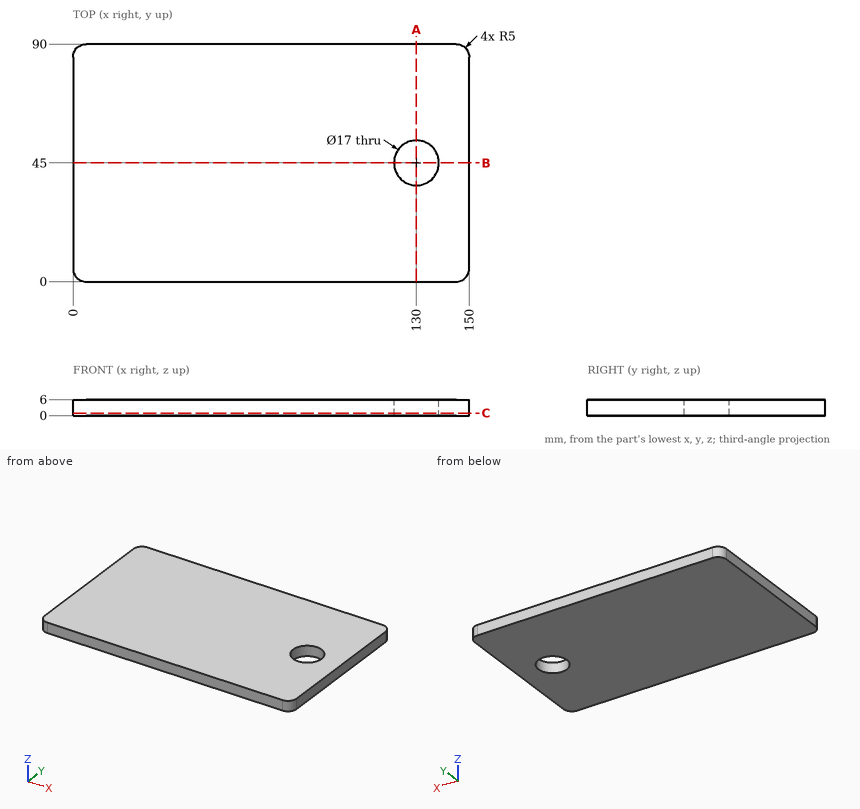
The figure shows three views and two pictorial views of one solid part (mm, origin at its lowest corner). Answer the questions. Give positions to 0.01 mm unless a question says otherwise; leave off trailing zeros. Write each loop counter-clockwise with the first axis right and the second up, starting at its lowest first coordinate (ties: lowest second). Pieces come first, ordered by that corner, then holes.
Q1. Given pin 1 (10 mm diameter, centred on x = 130, y = 45, fed in from +Z), flat-ended and moving along its own axis, determine where the tip first touches the part or whether it passes through.
Answer:
pin 1: passes through
Q2. Straight lines are drawn through the part: L1, parallel to Y at x = 130, z = 4.75; L2, parallel to X at y = 85.5, z = 3.8; L3, parallel to X at y = 44.5, z = 5. For each, find the intervals that lie inside material, in ascending order.
Answer:
L1: y = 0 to 36.5, 53.5 to 90
L2: x = 0.03 to 149.97
L3: x = 0 to 121.51, 138.49 to 150
Q3. The part is cut by section C-C on z = 0.9. Give the vertices of the cut face in (x, y).
Answer:
outline: (0, 5) arc R5 ccw to (5, 0) - (145, 0) arc R5 ccw to (150, 5) - (150, 85) arc R5 ccw to (145, 90) - (5, 90) arc R5 ccw to (0, 85) - close; hole circle Ø17 at (130, 45)
Q4. The part is cut by section B-B on y = 45. Give the vertices of the cut face in (x, z).
Answer:
outline: (0, 0) - (121.5, 0) - (121.5, 6) - (0, 6) - close; (138.5, 0) - (150, 0) - (150, 6) - (138.5, 6) - close
Q5. The part is cut by section A-A on x = 130. Give the vertices of the cut face in (y, z).
Answer:
outline: (0, 0) - (36.5, 0) - (36.5, 6) - (0, 6) - close; (53.5, 0) - (90, 0) - (90, 6) - (53.5, 6) - close
